Drawing for the job (mm, zero at the part's lowest x, y, z). Give positions to 0.01 mm unless a question says otherwise; leave off trailing zeros. Order: outer loops, then holes, each group sorted by start corner. A loop starts at its lowest first (then second) coordinate and runs counter-clockwise, first axis right, second up. Notation, with made-up numbers: (63, -23) - (104, -23) arc R25 cw to (104, -9) - close; hole circle Ø5 at (-21, -38). An arc over 180 degrees is marked (long way). Use a Markdown table: item, result.
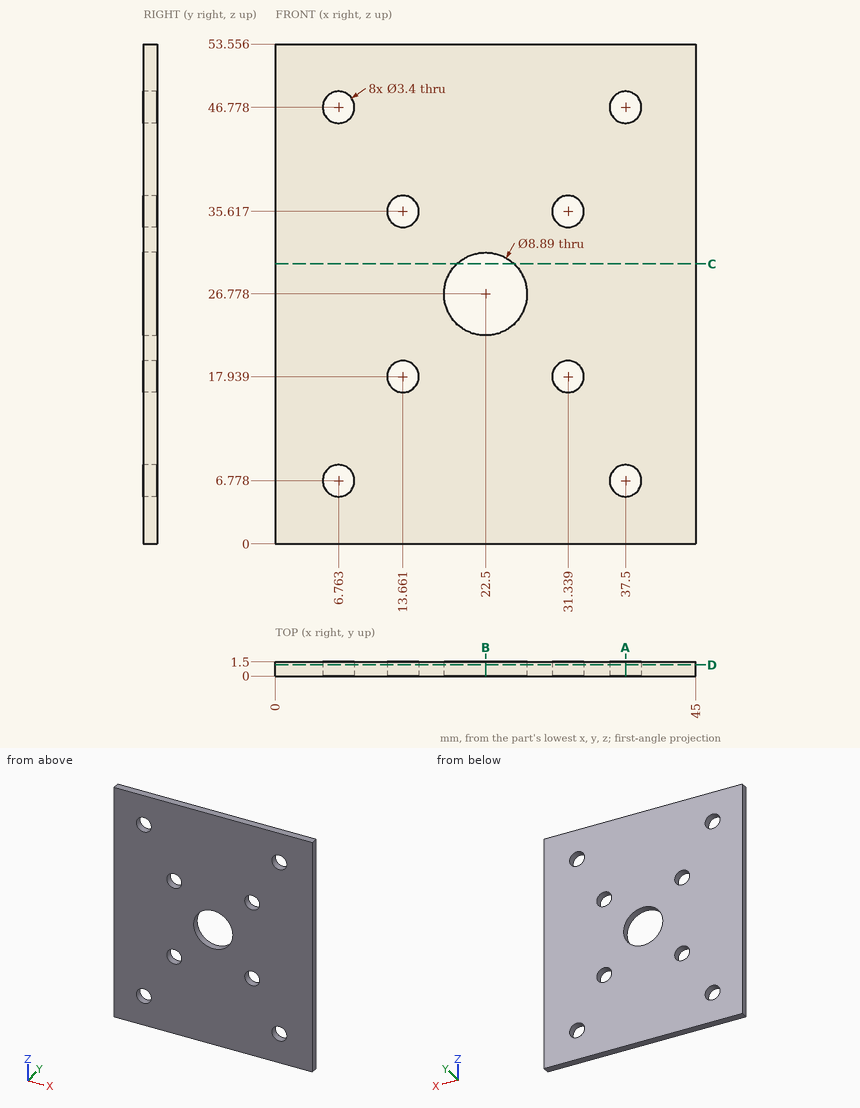
1) Wall check: line 1 (Z direction, x = 13.5, y = 0.65) (1 decimal); line 2 (X direction, y = 1.1, z = 47) (1 decimal); line 3 (X direction, y = 1.3, z = 27). Give the ranges that are in metal, low to high. Write a range as from..to.
Computed:
| item | result |
|---|---|
| line 1 | z = 0..16.2, 19.6..33.9, 37.3..53.6 |
| line 2 | x = 0..5.1, 8.4..35.8, 39.2..45 |
| line 3 | x = 0..18.06, 26.94..45 |
2) Slice it at D-D (y = 1.2). State how many separate pieces and enclosed holes the cut face has, and give its area (3 significant figures).
Computed:
| item | result |
|---|---|
| separate pieces | 1 |
| enclosed holes | 9 |
| area | 2,280 mm² |
3) Slice it at B-B (x = 22.5). Write the cut outline in (y, z).
Computed:
| item | result |
|---|---|
| outline | (0, 0) - (1.5, 0) - (1.5, 22.33) - (0, 22.33) - close; (0, 31.22) - (1.5, 31.22) - (1.5, 53.56) - (0, 53.56) - close |
4) Pin check, flat tip, straight feed: P1, Ø2.5, axis at x = 6.76, z = 6.78, coming from the -Y side. Stop position of the tip, or through.
Computed:
| item | result |
|---|---|
| P1 | passes through |
5) Slice it at C-C (z = 30). Write the cut outline in (x, y).
Computed:
| item | result |
|---|---|
| outline | (0, 0) - (19.44, 0) - (19.44, 1.5) - (0, 1.5) - close; (25.56, 0) - (45, 0) - (45, 1.5) - (25.56, 1.5) - close |
6) Slice it at A-A (x = 37.5). Write the cut outline in (y, z).
Computed:
| item | result |
|---|---|
| outline | (0, 0) - (1.5, 0) - (1.5, 5.08) - (0, 5.08) - close; (0, 8.48) - (1.5, 8.48) - (1.5, 45.08) - (0, 45.08) - close; (0, 48.48) - (1.5, 48.48) - (1.5, 53.56) - (0, 53.56) - close |
